CAD build for the part. Positions are in the model's coordinates, mm. A direction names the side the tool comes from. Give positions to 0.01 mm unless a question says otherwise; leave off trailing zeros. Write each loop counter-clockwise with the first axis right and the second up, starting at its lowest first coordinate (ties: lowest second). Pieces come first, ordered by that corner, then holes. Notation, with made-up numbers: (71, 26.5) -> (81, 26.5) arc R25 cw to (81, 39.5) -> close; hole circle Ø9 at (58, 69). An arc over 180 degrees is marked (long way). Answer as a JSON object with one key per item and string values.
```python
from build123d import *

# Parameters (mm, degrees)
BOSS_EXTRUDE1_DEPTH = 10
FILLET1_R           = 1
SKETCH3_R           = 2.25
CUT_EXTRUDE1_DEPTH  = 5


with BuildPart() as part:
    # Sketch2 → Boss-Extrude1 (new body)
    with BuildSketch(Plane.XY):
        with BuildLine():
            Line((-1.5, 9.9700831), (-1.5, 7.9700831))
            Line((-1.5, 7.9700831), (1.5, 7.9700831))
            Line((1.5, 7.9700831), (1.5, 6.3700831))
            Line((1.5, 6.3700831), (-8.5, 6.3700831))
            Line((-8.5, 6.3700831), (-8.5, 4.3700831))
            Line((-8.5, 4.3700831), (-4.933456572, 4.3700831))
            ThreePointArc((-4.933456572, 4.3700831), (-3.249951556, 3.449810315), (-3.115730388, 1.535893959))
            Line((-3.115730388, 1.535893959), (-7.463599773, -7.938259613))
            ThreePointArc((-7.463599773, -7.938259613), (-7.463263835, -9.607369524), (-6.197148301, -10.694972145))
            Line((-6.197148301, -10.694972145), (9.017188246, -15.057612947))
            Line((9.017188246, -15.057612947), (9.017188246, -12.456864357))
            Line((9.017188246, -12.456864357), (-0.280787764, -9.79071264))
            ThreePointArc((-0.280787764, -9.79071264), (-1.546903298, -8.703110018), (-1.547239236, -7.034000107))
            Line((-1.547239236, -7.034000107), (2.817726184, 2.4774063))
            ThreePointArc((2.817726184, 2.4774063), (2.953900249, 2.884660063), (3, 3.31159544))
            Line((3, 3.31159544), (3, 9.9700831))
            Line((3, 9.9700831), (-1.5, 9.9700831))
        make_face()
    extrude(amount=BOSS_EXTRUDE1_DEPTH)

    # Fillet1
    fillet1_edges = [part.edges().sort_by_distance(p)[0] for p in [
        (-8.5, 6.3700831, 5),
        (-1.5, 7.9700831, 5),
        (-1.5, 9.9700831, 5),
        (3, 9.9700831, 5),
        (-8.5, 4.3700831, 5),
    ]]
    fillet(fillet1_edges, radius=FILLET1_R - 0.0001)  # a hair under: the kernel refuses the full size

    # Sketch3 → Cut-Extrude1 (cut)
    with BuildSketch(Plane(origin=(-2.615476737, -9.121251349, 0), x_dir=(0.9612616959383208, -0.27563735581699245, 0), z_dir=(0.27563735581699245, 0.9612616959383208, 0))):
        with Locations(Location((7.101454819, -5, 0), (0, 0, 180))):
            Circle(SKETCH3_R)
    extrude(amount=-CUT_EXTRUDE1_DEPTH, mode=Mode.SUBTRACT)


solid = part.part
```
1) 3-axis set-ups, long thin cutter, end or side, ignore diameter. For faces 4 (the cylindrical face through (2.953, 2.879, 4.93)), 5 (the flat face through (-3, 6.37, 5)), 6 (the flat face through (-2, -2, 10)): which of +Z, -Z, +X, -X, +Y, -Y reach the whole face in a straight line?
Model answer:
{"face 4": "+Z, -Z, +X", "face 5": "+Z, -Z, -X", "face 6": "+Z, +X, -X, +Y, -Y"}
2) Pin check, flat tips, straight feed: pin 1 (0.6 mm diameter, centred on x = 0.5, z = 4.5, fed in from -Y); pin 2 (0.5 mm diameter, centred on y = 7, z = 3.5, fed in from -X); pin 3 (1.3 mm diameter, centred on x = -6, z = 6.5, fed in from -Y). Stop position of each tip, or through.
Model answer:
{"pin 1": "stops at y = -12.7", "pin 2": "stops at x = 1.5", "pin 3": "stops at y = -10.94"}
3) Slice it at B-B (x = 0.5). List the corners of the cut face in (y, z), then the cut area to 3 significant figures.
Model answer:
{"outline": "(-12.62, 0) -> (-10.01, 0) -> (-10.01, 10) -> (-12.62, 10) -> close; (-2.57, 0) -> (6.37, 0) -> (6.37, 10) -> (-2.57, 10) -> close; (7.97, 0) -> (9.97, 0) -> (9.97, 10) -> (7.97, 10) -> close", "area": "135 mm2"}
4) Wall check: probe 1 along Y at (x, z) = (0.75, 5.75); probe 2 along X at (y, z) = (9, 1.5); probe 3 along Y at (x, z) = (-1, 2.5). Give the ranges that are in metal, low to high.
Model answer:
{"probe 1": "y = -12.69 to -10.09, -2.03 to 6.37, 7.97 to 9.97", "probe 2": "x = -1.5 to 3", "probe 3": "y = -12.19 to -9.41, -5.84 to 6.37, 8.1 to 9.84"}
5) Slice it at D-D (y = -9.25). List the corners of the cut face in (x, z).
Model answer:
{"outline": "(-7.59, 0) -> (-1.18, 0) -> (-1.18, 10) -> (-7.59, 10) -> close"}
6) Mould opens along Y. For faces 1 (the cylindrical face through (2.715, 9.669, 5.07)), 2 (the cylindrical face through (-1.54, -8.72, 4.93)), 3 (the flat face through (1.304, -12.846, 3.819)) say: released by +Y, released by -Y, zero draft, split by the parting line, or undercut.
Model answer:
{"face 1": "released by +Y", "face 2": "undercut", "face 3": "released by -Y"}
